```python
from build123d import *

# Parameters (mm, degrees)
BOSS_EXTRUDE1_DEPTH = 14
CUT_EXTRUDE1_REACH  = 113.314
SKETCH4_R           = 2


with BuildPart() as part:
    # Sketch2 → Boss-Extrude1 (new body)
    with BuildSketch(Plane.XY):
        with BuildLine():
            Line((9.406636819, 3.393402975), (30.593363181, 3.393402975))
            Line((30.593363181, 3.393402975), (30.593363181, 18.393402975))
            Line((30.593363181, 18.393402975), (-109.406636819, 18.393402975))
            Line((-109.406636819, 18.393402975), (-109.406636819, 3.393402975))
            Line((-109.406636819, 3.393402975), (-9.406636819, 3.393402975))
            ThreePointArc((-9.406636819, 3.393402975), (0, 10), (9.406636819, 3.393402975))
        make_face()
    extrude(amount=BOSS_EXTRUDE1_DEPTH)

    # Sketch4 → Cut-Extrude1 (cut, up to next)
    with BuildSketch(Plane(origin=(0, 18.393402975, 0), x_dir=(1, 0, 0), z_dir=(0, 1, 0)), mode=Mode.PRIVATE) as cut_extrude1_sk1:
        with Locations(Location((20, -7, 0), (0, 0, 180))):
            Circle(SKETCH4_R)
    cut_extrude1_tool1 = extrude(cut_extrude1_sk1.sketch, amount=-CUT_EXTRUDE1_REACH, mode=Mode.PRIVATE) & part.part
    # Sketch4 → Cut-Extrude1 (cut, up to next)
    with BuildSketch(Plane(origin=(0, 18.393402975, 0), x_dir=(1, 0, 0), z_dir=(0, 1, 0)), mode=Mode.PRIVATE) as cut_extrude1_sk2:
        with Locations(Location((-20, -7, 0), (0, 0, 180))):
            Circle(SKETCH4_R)
    cut_extrude1_tool2 = extrude(cut_extrude1_sk2.sketch, amount=-CUT_EXTRUDE1_REACH, mode=Mode.PRIVATE) & part.part
    add(cut_extrude1_tool1.solids().sort_by_distance((20, 18.393403, 7))[0], mode=Mode.SUBTRACT)
    add(cut_extrude1_tool2.solids().sort_by_distance((-20, 18.393403, 7))[0], mode=Mode.SUBTRACT)


solid = part.part
```
Geometry check sheet. Reference: the model listing, model coordinates, mm. Give positions to 0.01 mm unless a question says otherwise; leave off trailing zeros. Order: outer loops, then holes, each group sorted by start corner. A loop starts at its lowest first (then second) coordinate and runs counter-clockwise, first axis right, second up. Notation, with made-up numbers: (70, -20.75) -> (117, -20.75) arc R35 cw to (117, 13.25) -> close; hole circle Ø8 at (33.5, 10). An arc over 180 degrees is marked (long way). Write each question's results on one line, items separated by ' | '. Start each with the question number.
(1) Sectioned sample at B-B (x = 20). Enter the section's corners in (y, z), plus the area to 3 significant figures.
(2) Gauge pin test, flat end, axial feed: P1, Ø3, axis at x = 20, z = 7, coming from the +Y side. Record the tip position at first contact, or that the pin passes through.
(3) Scan lines: line 1 (Z direction, x = -20, y = 14); line 2 (X direction, y = 13.5, z = 8.5); line 3 (X direction, y = 8.75, z = 12). Record each from-to range of solid material in increasing order.
(4) Mould release check, pull along Z, two halves, no side actions. Record for faces 1 (the face through (-40, 11, 14)), 2 (the face through (21.474, 10.998, 8.352)), 3 (the face through (-109.407, 11, 7)): pulls with the +Z half, pulls with the -Z half, needs draft (parallel to the pull), parting line crosses it, or undercut.
(5) Sectioned sample at A-A (z = 7). Enter the section's corners in (x, y), plus the area to 3 significant figures.
Answer below:
1) outline: (3.39, 0) -> (18.39, 0) -> (18.39, 5) -> (3.39, 5) -> close; (3.39, 9) -> (18.39, 9) -> (18.39, 14) -> (3.39, 14) -> close | area: 150 mm2
2) P1: through
3) line 1: 0 to 5, 9 to 14 | line 2: -109.41 to -21.32, -18.68 to 18.68, 21.32 to 30.59 | line 3: -109.41 to -4.84, 4.84 to 30.59
4) face 1: pulls with the +Z half | face 2: undercut | face 3: needs draft
5) outline: (-109.41, 3.39) -> (-22, 3.39) -> (-22, 18.39) -> (-109.41, 18.39) -> close; (-18, 3.39) -> (-9.41, 3.39) arc R10 cw to (9.41, 3.39) -> (18, 3.39) -> (18, 18.39) -> (-18, 18.39) -> close; (22, 3.39) -> (30.59, 3.39) -> (30.59, 18.39) -> (22, 18.39) -> close | area: 1,890 mm2
